Build history of the part. All positions in model axes, mm. Face numbers are marked on the shaded views. A direction names the side the tool comes from. Give positions to 0.01 mm unless a question says otherwise; leave off trailing zeros. Order: outer loops, then holes, each group sorted by start corner. A loop starts at its lowest first (then second) coordinate and runs counter-clockwise, first axis right, second up. Notation, with made-up numbers: (-23.5, 15) - (-10.5, 15) arc R31 cw to (-10.5, 45) - close; hole circle Ø4 at (65.5, 75.5). An arc over 180 degrees is marked (long way). Answer in a Markdown table with one row per item.
```python
from build123d import *

# Parameters (mm, degrees)
SKETCH1_R           = 18.5
SKETCH1_R_2         = 8.5
BOSS_EXTRUDE1_DEPTH = 8
SKETCH2_W           = 16
SKETCH2_H           = 53.319172682
BOSS_EXTRUDE2_DEPTH = 8
SKETCH3_W           = 16
SKETCH3_H           = 103.319172682
BOSS_EXTRUDE3_DEPTH = 8
SKETCH4_W           = 4
SKETCH4_H           = 2.038644179
CUT_EXTRUDE1_DEPTH  = 123.467342586
FILLET1_R           = 10
SKETCH7_R           = 6.5
CUT_EXTRUDE3_DEPTH  = 7
SKETCH8_R           = 3
CUT_EXTRUDE4_DEPTH  = 122.750770018
SKETCH9_R           = 3
CUT_EXTRUDE5_DEPTH  = 124.151329672


with BuildPart() as part:
    # Sketch1 → Boss-Extrude1 (new, symmetric)
    with BuildSketch(Plane.XY):
        Circle(SKETCH1_R)
        Circle(SKETCH1_R_2, mode=Mode.SUBTRACT)
    extrude(amount=BOSS_EXTRUDE1_DEPTH, both=True)

    # Sketch2 → Boss-Extrude2 (add, symmetric)
    with BuildSketch(Plane.XY):
        with Locations((0, 43.340413659)):
            Rectangle(SKETCH2_W, SKETCH2_H)
    extrude(amount=BOSS_EXTRUDE2_DEPTH, both=True)

    # Sketch3 → Boss-Extrude3 (add, symmetric)
    with BuildSketch(Plane.XY):
        with Locations((0, -68.340413659)):
            Rectangle(SKETCH3_W, SKETCH3_H)
    extrude(amount=BOSS_EXTRUDE3_DEPTH, both=True)

    # Sketch4 → Cut-Extrude1 (cut, through all)
    with BuildSketch(Plane(origin=(0, 0, -8), x_dir=(-1, 0, 0), z_dir=(0, 0, -1))):
        with Locations((0, 9.28067791)):
            Rectangle(SKETCH4_W, SKETCH4_H)
    extrude(amount=-CUT_EXTRUDE1_DEPTH, mode=Mode.SUBTRACT)

    # Fillet1
    fillet1_edges = [part.edges().sort_by_distance(p)[0] for p in [
        (8, 16.680827318, 0),
        (-8, 16.680827318, 0),
        (8, -16.680827318, 0),
        (-8, -16.680827318, 0),
    ]]
    fillet(fillet1_edges, radius=FILLET1_R)

    # Sketch7 → Cut-Extrude3 (cut)
    with BuildSketch(Plane.XY.offset(8)):
        with Locations((0, 55)):
            Circle(SKETCH7_R)
        with Locations((0, 30)):
            Circle(SKETCH7_R)
    cut_extrude3 = extrude(amount=-CUT_EXTRUDE3_DEPTH, mode=Mode.SUBTRACT)

    # Mirror1: Cut-Extrude3 across plane
    add(cut_extrude3.mirror(Plane.ZX), mode=Mode.SUBTRACT)

    # Sketch8 → Cut-Extrude4 (cut, through all)
    with BuildSketch(Plane.XY.offset(1)):
        with Locations((0, 55)):
            Circle(SKETCH8_R)
        with Locations((0, 30)):
            Circle(SKETCH8_R)
    cut_extrude4 = extrude(amount=-CUT_EXTRUDE4_DEPTH, mode=Mode.SUBTRACT)

    # Mirror2: Cut-Extrude4 across plane
    add(cut_extrude4.mirror(Plane.ZX), mode=Mode.SUBTRACT)

    # Sketch9 → Cut-Extrude5 (cut, through all)
    with BuildSketch(Plane(origin=(8, 0, 0), x_dir=(0, 0, -1), z_dir=(1, 0, 0))):
        with Locations(Location((0, -110, 0), (0, 0, 90))):
            Circle(SKETCH9_R)
        with Locations(Location((0, -90, 0), (0, 0, 90))):
            Circle(SKETCH9_R)
    extrude(amount=-CUT_EXTRUDE5_DEPTH, mode=Mode.SUBTRACT)


solid = part.part
```
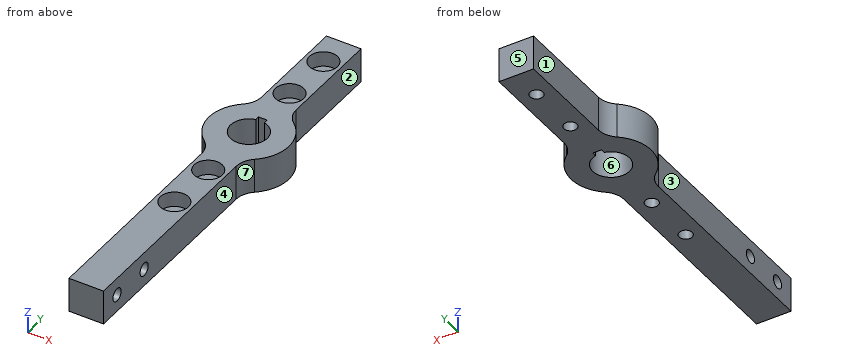
1. Drop flat-ended pins along their axis: P1, Ø8, axis at y = -90, z = 0, coming from the -X side; P2, Ø3.5, axis at x = 0, y = -55, coming from the +Z side; P3, Ø6, axis at x = 12, z = 2, coming from the -Y side; P4, Ø8, axis at y = -68.5, z = 0.5, coming from the +X side. Give the stop position or say it passes through.
Check result:
| item | result |
|---|---|
| P1 | stops at x = -8 |
| P2 | passes through |
| P3 | stops at y = -17.74 |
| P4 | stops at x = 8 |
2. Cut at C-C on z = -5.75. Write the cut outline in (x, y).
Check result:
| item | result |
|---|---|
| outline | (-11.68, -14.34) arc R10 cw to (-8, -22.1) - (-8, -120) - (8, -120) - (8, -22.1) arc R10 cw to (11.68, -14.34) arc R18.5 ccw to (11.68, 14.34) arc R10 cw to (8, 22.1) - (8, 70) - (-8, 70) - (-8, 22.1) arc R10 cw to (-11.68, 14.34) arc R18.5 ccw to start; hole circle Ø6 at (0, -55); hole circle Ø6 at (0, -30); hole circle Ø6 at (0, 30); hole circle Ø6 at (0, 55); hole (-2, 8.26) arc R8.5 ccw (long way) to (2, 8.26) - (2, 10.3) - (-2, 10.3) - close |
3. Two-plate mould, pull along Y, no slides. Class the marked faces 5, 6 and 7: +Y half, -Y half, draft (parallel to the pull), parting line (faces both ways), or undercut.
Check result:
| item | result |
|---|---|
| face 5 | +Y half |
| face 6 | undercut |
| face 7 | -Y half |
4. Which spindle directions (+Z, -Z, +X, -X, +Y, -Y) get a long thin tool onto all of the face, cutting with end or side? Do the marked faces 1, 2, 3 and 4. Say none if no direction does.
Check result:
| item | result |
|---|---|
| face 1 | +Z, -Z, -X, +Y |
| face 2 | +Z, -Z, +X, +Y |
| face 3 | +Z, -Z, -X, -Y |
| face 4 | +Z, -Z, +X, -Y |
5. Probe line 1 (Y direction, x = 0, z = 3.25); line 2 (Y direction, x = -2.5, z = -4.25); line 3 (Z direction, x = -3, y = -110). List the from-to ranges inside material, lowest first.
Check result:
| item | result |
|---|---|
| line 1 | y = -120 to -61.5, -48.5 to -36.5, -23.5 to -8.5, 10.3 to 23.5, 36.5 to 48.5, 61.5 to 70 |
| line 2 | y = -120 to -56.66, -53.34 to -31.66, -28.34 to -8.12, 8.12 to 28.34, 31.66 to 53.34, 56.66 to 70 |
| line 3 | z = -8 to -3, 3 to 8 |
6. Cut at B-B on x = 0. Count the separate pieces of the cut face and the enclosed holes in it, and give its area (3 significant figures).
Check result:
| item | result |
|---|---|
| separate pieces | 6 |
| enclosed holes | 2 |
| area | 2,100 mm² |
7. Cut at D-D on y = -90. Write the cut outline in (x, z).
Check result:
| item | result |
|---|---|
| outline | (-8, -8) - (8, -8) - (8, -3) - (-8, -3) - close; (-8, 3) - (8, 3) - (8, 8) - (-8, 8) - close |
8. Cut at A-A on y = 0. Write the cut outline in (x, z).
Check result:
| item | result |
|---|---|
| outline | (-18.5, -8) - (-8.5, -8) - (-8.5, 8) - (-18.5, 8) - close; (8.5, -8) - (18.5, -8) - (18.5, 8) - (8.5, 8) - close |
